from build123d import *

# Parameters (mm, degrees)
CROQUIS1_R              = 2.75
SALIENTE_EXTRUIR1_DEPTH = 5
CROQUIS3_R              = 5
CROQUIS3_R_2            = 2.75
SALIENTE_EXTRUIR2_DEPTH = 6
CROQUIS2_R              = 0.75
CORTAR_EXTRUIR1_DEPTH   = 15.508806178


with BuildPart() as part:
    # Croquis1 → Saliente-Extruir1 (new body)
    with BuildSketch(Plane(origin=(0, 0, 0), x_dir=(1, 0, 0), z_dir=(0, 1, 0))):
        Polygon((1.401704423, 6.784926286), (-5.175066315, 4.606374782), (-6.576770738, -2.178551504), (-1.401704423, -6.784926286), (5.175066315, -4.606374782), (6.576770738, 2.178551504), align=None)
        Circle(CROQUIS1_R, mode=Mode.SUBTRACT)
    extrude(amount=SALIENTE_EXTRUIR1_DEPTH)

    # Croquis3 → Saliente-Extruir2 (add)
    with BuildSketch(Plane(origin=(0, 5, 0), x_dir=(1, 0, 0), z_dir=(0, 1, 0))):
        Circle(CROQUIS3_R)
        Circle(CROQUIS3_R_2, mode=Mode.SUBTRACT)
    extrude(amount=SALIENTE_EXTRUIR2_DEPTH)

    # Croquis2 → Cortar-Extruir1 (cut, through all)
    with BuildSketch(Plane(origin=(1.886680946, 0, 5.695650534), x_dir=(0.949275089, 0, -0.314446824), z_dir=(0.314446824, 0, 0.949275089))):
        with Locations((0, 1.5)):
            Circle(CROQUIS2_R)
    extrude(amount=-CORTAR_EXTRUIR1_DEPTH, mode=Mode.SUBTRACT)


solid = part.part
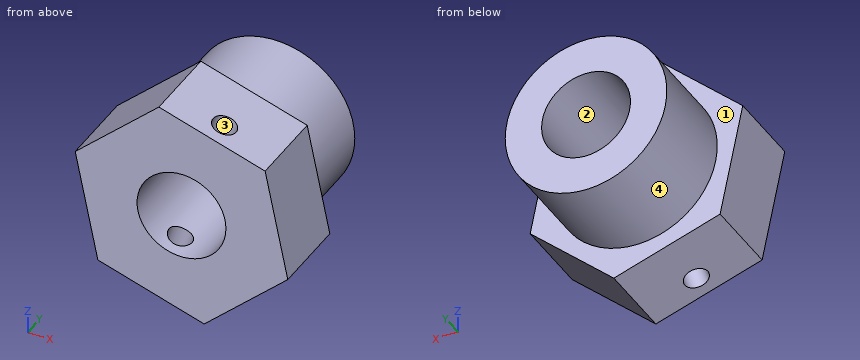
The listing builds one solid part. Answer for the finished solid, in the listing's coordinates (mm). Face numbers are marked on the shaded views. Coordinates: 2 decimals unless noted, no trailing zeros. Write each loop counter-clockwise with the first axis right and the second up, starting at its lowest first coordinate (ties: lowest second). Pieces come first, ordered by that corner, then holes. Notation, with made-up numbers: M -9,-31.5 L 7,-31.5 A36 cw 7,5.5 Z; hole C 40.5,49.25 d2. An arc over 180 degrees is marked long. Write each question's results on one line, items separated by ' | '.
Item 1: The part is cut by section A-A on z = -1.75. Determine the outline of the cut face in (x, y).
Answer below:
outline: M -5.77,0 L -2.12,0 L -2.12,11 L -4.68,11 L -4.68,5 L -5.77,5 Z; M 2.12,0 L 6.49,0 L 6.49,5 L 4.68,5 L 4.68,11 L 2.12,11 Z
Item 2: The part is cut by section C-C on y = 10.5. Determine the outline of the cut face in (x, z), and give its area (3 significant figures).
Answer below:
outline: C 0,0 d10; hole C 0,0 d5.5 | area: 54.8 mm2
Item 3: The part is cut by section D-D on z = 0. Determine the outline of the cut face in (x, y).
Answer below:
outline: M -6.13,0 L -2.75,0 L -2.75,11 L -5,11 L -5,5 L -6.13,5 Z; M 2.75,0 L 6.13,0 L 6.13,5 L 5,5 L 5,11 L 2.75,11 Z
Item 4: Given P1, Ø4, axis at y = 4.5, z = 2.5, coming from the +X side; P2, Ø2, axis at y = 5.5, z = -3, coming from the -X side; P3, Ø6, axis at x = 0, y = 1.5, coming from the +Z side; P4, Ø2, axis at y = 9, z = 3.5, coming from the -X side, each flat-ended and moving along its own axis, determine where each tip first touches the part or whether it passes through.
Answer below:
P1: x = 6.02 | P2: x = -5.69 | P3: z = 6.78 | P4: x = -4.33
Item 5: Consider probe 1 along Z at (x, y) = (0, 8.25); probe 2 along Z at (x, y) = (0, 2.5). Determine where each line is inside the solid, lowest interval first. Write a range as [from, to].
Answer below:
probe 1: [-5, -2.75], [2.75, 5] | probe 2: [-6.32, -2.75], [2.75, 6.32]
Item 6: For a pull along X with two mould halves and no side action, classify the marked faces 1, 2, 3 and 4 as released by +X, released by -X, zero draft, split by the parting line, or undercut.
Answer below:
face 1: zero draft | face 2: undercut | face 3: undercut | face 4: split by the parting line
Item 7: The part is cut by section B-B on x = 4.5. Determine the outline of the cut face in (y, z).
Answer below:
outline: M 0,-4.03 L 5,-4.03 L 5,-2.18 L 11,-2.18 L 11,2.18 L 5,2.18 L 5,4.83 L 0,4.83 Z
